The listing builds one solid part. Answer for the finished solid, in the listing's coordinates (mm). A direction names the side the tool comes from. Coordinates: 2 decimals unless noted, no trailing zeros. Order: outer loops, then holes, each group sorted by start corner. A loop starts at its lowest first (then second) coordinate and runs counter-clockwise, first axis right, second up. Notation, with made-up numbers: (-2.5, 27.5) -> (27.5, 27.5) arc R24 cw to (27.5, 38.5) -> close; hole circle Ø5 at (-12.75, 80.5). An arc over 180 degrees is marked (long way). Answer in a Markdown table with one row per item.
```python
from build123d import *

# Parameters (mm, degrees)
SKETCH1_W           = 19.05
SKETCH1_H           = 47
BOSS_EXTRUDE1_DEPTH = 2.54
SKETCH2_R           = 8.44
BOSS_EXTRUDE2_DEPTH = 3
SKETCH3_R           = 1.5
CUT_EXTRUDE1_DEPTH  = 56.204627156


with BuildPart() as part:
    # Sketch1 → Boss-Extrude1 (new body)
    with BuildSketch(Plane(origin=(0, 0, 0), x_dir=(1, 0, 0), z_dir=(0, 1, 0))):
        with Locations((9.525, 23.5)):
            Rectangle(SKETCH1_W, SKETCH1_H)
    extrude(amount=BOSS_EXTRUDE1_DEPTH)

    # Sketch2 → Boss-Extrude2 (add)
    with BuildSketch(Plane.ZY):
        with BuildLine():
            Line((-23.526869674, 17.516472082), (-23.473130326, 17.516472082))
            ThreePointArc((-23.473130326, 17.516472082), (-20.760886981, 18.164487773), (-18.634502385, 19.968560069))
            ThreePointArc((-18.634502385, 19.968560069), (-8.591509803, 24.257746253), (0, 17.516472082))
            Line((0, 17.516472082), (0, 2.54))
            Line((0, 2.54), (-47, 2.54))
            Line((-47, 2.54), (-47, 17.516472082))
            ThreePointArc((-47, 17.516472082), (-38.408490197, 24.257746253), (-28.365497615, 19.968560069))
            ThreePointArc((-28.365497615, 19.968560069), (-26.239113019, 18.164487773), (-23.526869674, 17.516472082))
        make_face()
        with Locations((-9.99, 13.63)):
            Circle(SKETCH2_R, mode=Mode.SUBTRACT)
        with Locations((-37.01, 13.63)):
            Circle(SKETCH2_R, mode=Mode.SUBTRACT)
    extrude(amount=-BOSS_EXTRUDE2_DEPTH)

    # Sketch3 → Cut-Extrude1 (cut, through all)
    with BuildSketch(Plane(origin=(0, 2.54, 0), x_dir=(1, 0, 0), z_dir=(0, 1, 0))):
        with Locations(Location((15.274497475, 10.68388452, 0), (0, 0, 270))):
            Circle(SKETCH3_R)
        with Locations(Location((15.33, 36.095973984, 0), (0, 0, 270))):
            Circle(SKETCH3_R)
    extrude(amount=-CUT_EXTRUDE1_DEPTH, mode=Mode.SUBTRACT)


solid = part.part
```
(1) For a pull along Y with two mould halves and no side action, classify faces 1 (the cylindrical face through (1.479, 20.747, -32.473)), 2 (the cylindrical face through (1.479, 24.277, -8.751)), 3 (the cylindrical face through (1.479, 20.747, -5.453)), 4 (the flat face through (0, 10, -23)) as released by +Y, released by -Y, zero draft, split by the parting line, or undercut.
Check values:
| item | result |
|---|---|
| face 1 | undercut |
| face 2 | released by +Y |
| face 3 | undercut |
| face 4 | zero draft |
(2) A cutting plane is placed at B-B, the plane z = -9.99. Determine the outline of the cut face in (x, y), then the cut area to 3 significant figures.
Check values:
| item | result |
|---|---|
| outline | (0, 0) -> (13.94, 0) -> (13.94, 2.54) -> (3, 2.54) -> (3, 5.19) -> (0, 5.19) -> close; (0, 22.07) -> (3, 22.07) -> (3, 24.35) -> (0, 24.35) -> close; (16.6, 0) -> (19.05, 0) -> (19.05, 2.54) -> (16.6, 2.54) -> close |
| area | 56.4 mm² |
(3) Flat-ended cylindrical pins translate along their axes: pin 1 (2 mm diameter, centred on y = 20, z = -11, fed in from +X); pin 2 (2 mm diameter, centred on x = 10, z = -35, fed in from +Y); pin 3 (1 mm diameter, centred on y = 13.5, z = -20, fed in from +X). Find the tip coordinate at first contact, or state that the pin passes through.
Check values:
| item | result |
|---|---|
| pin 1 | through |
| pin 2 | y = 2.54 |
| pin 3 | x = 3 |
(4) A cutting plane is placed at D-D, the plane x = 8.5. Determine the outline of the cut face in (y, z).
Check values:
| item | result |
|---|---|
| outline | (0, -47) -> (2.54, -47) -> (2.54, 0) -> (0, 0) -> close |
(5) Which of the six approach directions +Z, -Z, +X, -X, +Y, -Y give full straight-line access (tool end or side, diameter ignored) to faces 5 (the flat face through (11, 2.54, -24)), 6 (the cylindrical face through (1.48, 18.18, -26.27)), 7 (the flat face through (5, 2, -47))?
Check values:
| item | result |
|---|---|
| face 5 | +Z, -Z, +X, +Y |
| face 6 | +X, -X, +Y |
| face 7 | -Z, +X, -X, +Y, -Y |
(6) A cutting plane is placed at A-A, the plane y = 13.63. Determine the outline of the cut face in (x, z), then the cut area to 3 significant figures.
Check values:
| item | result |
|---|---|
| outline | (0, -47) -> (3, -47) -> (3, -45.45) -> (0, -45.45) -> close; (0, -28.57) -> (3, -28.57) -> (3, -18.43) -> (0, -18.43) -> close; (0, -1.55) -> (3, -1.55) -> (3, 0) -> (0, 0) -> close |
| area | 39.7 mm² |
(7) A cutting plane is placed at C-C, the plane y = 20.5. Determine the outline of the cut face in (x, z).
Check values:
| item | result |
|---|---|
| outline | (0, -45.24) -> (3, -45.24) -> (3, -41.91) -> (0, -41.91) -> close; (0, -32.11) -> (3, -32.11) -> (3, -28.78) -> (0, -28.78) -> close; (0, -18.22) -> (3, -18.22) -> (3, -14.89) -> (0, -14.89) -> close; (0, -5.09) -> (3, -5.09) -> (3, -1.76) -> (0, -1.76) -> close |
(8) Find the intervals of material crossed by line 1 along Y through (x, z) = (0.7, -37.01); line 2 along Y through (x, z) = (5.75, -44); line 3 along Y through (x, z) = (1.5, -40), in increasing order. Write a range as from..to.
Check values:
| item | result |
|---|---|
| line 1 | 0..5.19, 22.07..24.35 |
| line 2 | 0..2.54 |
| line 3 | 0..5.74, 21.52..23.92 |
